```python
from build123d import *

# Parameters (mm, degrees)
SKETCH1_W                       = 30
SKETCH1_H                       = 20
BOSS_EXTRUDE1_DEPTH             = 4
SKETCH2_W                       = 20
SKETCH2_H                       = 20
BOSS_EXTRUDE2_DEPTH             = 4
CBORE_FOR_M5_SBHCS1_D           = 5.5
CBORE_FOR_M5_SBHCS1_CBORE_D     = 9
CBORE_FOR_M5_SBHCS1_CBORE_DEPTH = 1
SKETCH10_W                      = 10
SKETCH10_H                      = 4
BOSS_EXTRUDE3_DEPTH             = 50
BOSS_EXTRUDE4_DEPTH             = 15
SKETCH11_W                      = 10
SKETCH11_H                      = 13
BOSS_EXTRUDE5_DEPTH             = 2
SKETCH12_R                      = 1
CUT_EXTRUDE1_DEPTH              = 4
CHAMFER1_SIZE                   = 1.5


with BuildPart() as part:
    # Sketch1 → Boss-Extrude1 (new body)
    with BuildSketch(Plane(origin=(0, 0, 0), x_dir=(1, 0, 0), z_dir=(0, 1, 0))):
        with Locations((15, 10)):
            Rectangle(SKETCH1_W, SKETCH1_H)
    extrude(amount=BOSS_EXTRUDE1_DEPTH)

    # Sketch2 → Boss-Extrude2 (add)
    with BuildSketch(Plane.XZ):
        with Locations((10, -10)):
            Rectangle(SKETCH2_W, SKETCH2_H)
    extrude(amount=BOSS_EXTRUDE2_DEPTH)

    # CBORE for M5 SBHCS1 (through all)
    with Locations(Plane(origin=(0, 4, 0), x_dir=(1, 0, 0), z_dir=(0, 1, 0))):
        with Locations((10, 10)):
            CounterBoreHole(CBORE_FOR_M5_SBHCS1_D / 2, CBORE_FOR_M5_SBHCS1_CBORE_D / 2, CBORE_FOR_M5_SBHCS1_CBORE_DEPTH)

    # Sketch10 → Boss-Extrude3 (add)
    with BuildSketch(Plane(origin=(0, 0, -20), x_dir=(-1, 0, 0), z_dir=(0, 0, -1))):
        with Locations((-25, 2)):
            Rectangle(SKETCH10_W, SKETCH10_H)
    extrude(amount=BOSS_EXTRUDE3_DEPTH)

    # Sketch10<3> → Boss-Extrude4 (add)
    with BuildSketch(Plane(origin=(0, 0, -20), x_dir=(-1, 0, 0), z_dir=(0, 0, -1))):
        Polygon((-18.5, 4), (-20, 4), (-20, 0), (-20, -1.5), (-18.5, -1.5), align=None)
    extrude(amount=BOSS_EXTRUDE4_DEPTH)

    # Sketch11 → Boss-Extrude5 (add)
    with BuildSketch(Plane(origin=(0, 4, 0), x_dir=(1, 0, 0), z_dir=(0, 1, 0))):
        with Locations((25, 63.5)):
            Rectangle(SKETCH11_W, SKETCH11_H)
    extrude(amount=BOSS_EXTRUDE5_DEPTH)

    # Sketch12 → Cut-Extrude1 (cut)
    with BuildSketch(Plane(origin=(0, 6, 0), x_dir=(1, 0, 0), z_dir=(0, 1, 0))):
        with Locations(Location((28, 60.25, 0), (0, 0, 270))):
            Circle(SKETCH12_R)
        with Locations(Location((28, 66.75, 0), (0, 0, 270))):
            Circle(SKETCH12_R)
    extrude(amount=-CUT_EXTRUDE1_DEPTH, mode=Mode.SUBTRACT)

    # Chamfer1
    chamfer1_edges = [part.edges().sort_by_distance(p)[0] for p in [
        (20, 2, -35),
    ]]
    chamfer(chamfer1_edges, length=CHAMFER1_SIZE - 0.0001)  # a hair under: the kernel refuses the full size


solid = part.part
```
Model file for the job. Use its own axes, mm. A direction names the side the tool comes from. Coordinates: 2 decimals unless noted, no trailing zeros. Write each loop counter-clockwise with the first axis right and the second up, starting at its lowest first coordinate (ties: lowest second). Pieces come first, ordered by that corner, then holes. Notation, with made-up numbers: (33.25, 23.5) - (86.25, 23.5) arc R24 cw to (86.25, 46.5) - close; hole circle Ø6 at (27, -36.75). An arc over 180 degrees is marked (long way). One line per item, written item: value. Start each with the question number.
1. Slice it at B-B (x = 10). Write the cut outline in (y, z).
2. Flat gauge pins, fed straight in: pin 1 (1.8 mm diameter, centred on y = 2.5, z = -47.5, fed in from -X); pin 2 (1.2 mm diameter, centred on y = -1.5, z = -18.5, fed in from +X); pin 3 (4.5 mm diameter, centred on x = 10, z = -8, fed in from +Y). Where does each tip first touch, or does it go through?
3. Slice it at C-C (y = -2.25). Write the cut outline in (x, z).
4. Slice it at A-A (z = -10). Write the cut outline in (x, y).
5. Probe line 1 (Z direction, x = 10, y = 3.75); line 2 (X direction, y = 0.5, z = -10); line 3 (Z direction, x = 16.25, y = -1.5). List the from-to ranges inside material, lowest first. Write a range as from..to.
6. Slice it at D-D (x = 28). Write the cut outline in (y, z), plus the area to 3 significant figures.
7. Tool access for faces 1 (the flat face through (18.5, 1, -27)), 2 (the flat face through (25, 5, -57)), 3 (the flat face through (19, -1, -35)), 4 (the flat face through (28, 2, -67)): list every direction of +Z, -Z, +X, -X, +Y, -Y with a clear straight run to the whole face (end or side of a thin tool).
8. Mould opens along Z. For faces 5 (the flat face through (19.2, 2, -35.7)), 6 (the flat face through (19, -1.5, -27)), 7 (the cylindrical face through (28.676, 4.028, -60.987)) say: released by +Z, released by -Z, zero draft, split by the parting line, or undercut.
Answers below:
1. outline: (-4, -20) - (4, -20) - (4, -14.5) - (3, -14.5) - (3, -12.75) - (-4, -12.75) - close; (-4, -7.25) - (3, -7.25) - (3, -5.5) - (4, -5.5) - (4, 0) - (-4, 0) - close
2. pin 1: stops at x = 20
2. pin 2: stops at x = 20
2. pin 3: stops at y = 3
3. outline: (0, -20) - (20, -20) - (20, 0) - (0, 0) - close; hole circle Ø5.5 at (10, -10)
4. outline: (0, -4) - (7.25, -4) - (7.25, 3) - (5.5, 3) - (5.5, 4) - (0, 4) - close; (12.75, -4) - (20, -4) - (20, 0) - (30, 0) - (30, 4) - (14.5, 4) - (14.5, 3) - (12.75, 3) - close
5. line 1: z = -20..-14.5, -5.5..0
5. line 2: x = 0..7.25, 12.75..30
5. line 3: z = -20..0
6. outline: (0, -70) - (6, -70) - (6, -67.75) - (2, -67.75) - (2, -65.75) - (6, -65.75) - (6, -61.25) - (2, -61.25) - (2, -59.25) - (6, -59.25) - (6, -57) - (4, -57) - (4, 0) - (0, 0) - close
6. area: 290 mm^2
7. face 1: -Z, -X, +Y, -Y
7. face 2: +Z, +X, -X, +Y
7. face 3: -Z, +X, -X, -Y
7. face 4: +Y
8. face 5: released by -Z
8. face 6: zero draft
8. face 7: undercut
